Check sheet for the modelled part. Datum: model origin and axes. Units: mm. Face numbers are marked on the shaded views. A direction names the side the tool comes from. Give positions to 0.01 mm unless a question says otherwise; leave off trailing zeros. Loops run counter-clockwise (first coordinate to the right, second up) from the corner with the lowest first, then second, coordinate; pieces in that order, holes last. Notation, with made-up numbers: M 17,45 L 70,45 A16 ccw 70,71 Z; hole C 25,79.25 d1. An arc over 180 degrees is marked long. One line per question, with ' | ' between items. Start each with the question number.
from build123d import *

# Parameters (mm, degrees)
SKETCH1_W           = 30.4
SKETCH1_H           = 3.2
BOSS_EXTRUDE1_DEPTH = 17.6
SKETCH2_R           = 1.5
CUT_EXTRUDE1_DEPTH  = 16
SKETCH3_R           = 1.075
CUT_EXTRUDE2_DEPTH  = 16
SKETCH4_W           = 22.4
SKETCH4_H           = 3.2
BOSS_EXTRUDE2_DEPTH = 12.8
SKETCH5_R           = 1.075
CUT_EXTRUDE3_DEPTH  = 16
SKETCH6_W           = 14.4
SKETCH6_H           = 14.4
BOSS_EXTRUDE3_DEPTH = 3.2
SKETCH7_R           = 1.5
CUT_EXTRUDE4_DEPTH  = 59.356147919
SKETCH8_R           = 6
CUT_EXTRUDE5_DEPTH  = 3.2
FILLET5_R           = 4
FILLET6_R           = 10
FILLET7_R           = 6
FILLET8_R           = 10
FILLET9_R           = 3
FILLET10_R          = 10
FILLET12_R          = 3


# Some blends are built 0.0001 mm under size
with BuildPart() as part:
    # Sketch1 → Boss-Extrude1 (new body)
    with BuildSketch(Plane(origin=(0, 0, 0), x_dir=(1, 0, 0), z_dir=(0, 1, 0))):
        with Locations((15.2, -1.6)):
            Rectangle(SKETCH1_W, SKETCH1_H)
    extrude(amount=BOSS_EXTRUDE1_DEPTH)

    # Sketch2 → Cut-Extrude1 (cut)
    with BuildSketch(Plane.XY.offset(3.2)):
        with Locations((23.2, 6.4)):
            Circle(SKETCH2_R)
        with Locations((7.2, 6.4)):
            Circle(SKETCH2_R)
    extrude(amount=-CUT_EXTRUDE1_DEPTH, mode=Mode.SUBTRACT)

    # Sketch3 → Cut-Extrude2 (cut)
    with BuildSketch(Plane(origin=(0, 0, 0), x_dir=(-1, 0, 0), z_dir=(0, 0, -1))):
        with Locations((-27.2, 12.8)):
            Circle(SKETCH3_R)
        with Locations((-3.2, 12.8)):
            Circle(SKETCH3_R)
    extrude(amount=-CUT_EXTRUDE2_DEPTH, mode=Mode.SUBTRACT)

    # Sketch4 → Boss-Extrude2 (add)
    with BuildSketch(Plane(origin=(0, 17.6, 0), x_dir=(1, 0, 0), z_dir=(0, 1, 0))):
        with Locations((15.2, -1.6)):
            Rectangle(SKETCH4_W, SKETCH4_H)
    extrude(amount=BOSS_EXTRUDE2_DEPTH)

    # Sketch5 → Cut-Extrude3 (cut)
    with BuildSketch(Plane.XY.offset(3.2)):
        with Locations((12, 24)):
            Circle(SKETCH5_R)
    extrude(amount=-CUT_EXTRUDE3_DEPTH, mode=Mode.SUBTRACT)

    # Sketch6 → Boss-Extrude3 (add)
    with BuildSketch(Plane.XY.offset(3.2)):
        with Locations((-3.2, 34.4)):
            Rectangle(SKETCH6_W, SKETCH6_H)
        with Locations((33.6, 34.4)):
            Rectangle(SKETCH6_W, SKETCH6_H)
    extrude(amount=-BOSS_EXTRUDE3_DEPTH)

    # Sketch7 → Cut-Extrude4 (cut, through all)
    with BuildSketch(Plane.XY.offset(3.2)):
        with Locations((-6.725, 38.2)):
            Circle(SKETCH7_R)
        with Locations((37.125, 38.2)):
            Circle(SKETCH7_R)
    extrude(amount=-CUT_EXTRUDE4_DEPTH, mode=Mode.SUBTRACT)

    # Sketch8 → Cut-Extrude5 (cut)
    with BuildSketch(Plane.XY.offset(3.2)):
        with Locations((15.2, 35.549818305)):
            Circle(SKETCH8_R)
    extrude(amount=-CUT_EXTRUDE5_DEPTH, mode=Mode.SUBTRACT)

    # Fillet5
    fillet5_edges = [part.edges().sort_by_distance(p)[0] for p in [
        (0, 17.6, 1.6),
        (30.4, 17.6, 1.6),
    ]]
    fillet(fillet5_edges, radius=FILLET5_R - 0.0001)  # a hair under: the kernel refuses the full size

    # Fillet6
    # the kernel refuses this fillet: 10 mm, written as the material it adds along each edge
    with BuildSketch(Plane(origin=(26.4, 30.4, 3.2), x_dir=(0, 1, 0), z_dir=(0, 0, -1)), Plane(origin=(4, 30.4, 0), x_dir=(0, 1, 0), z_dir=(0, 0, 1))) as fillet6_piece_1:
        with BuildLine():
            CenterArc((9.821908657, -10), FILLET6_R, 90, 79.170567871)
            Line((0, -8.121141214), (-0.196438173, -8.083564039))
            ThreePointArc((-0.196438173, -8.083564039), (-0.2, -4.060570607), (-0.2, 0))
            Line((-0.2, 0), (0, 0.2))
            Line((0, 0.2), (9.821908657, 0.2))
            Line((9.821908657, 0.2), (9.821908657, 0))
        make_face()
    extrude(amount=3.2)

    # Fillet7
    fillet7_edges = [part.edges().sort_by_distance(p)[0] for p in [
        (4, 27.2, 1.6),
        (26.4, 27.2, 1.6),
    ]]
    fillet(fillet7_edges, radius=FILLET7_R)

    # Fillet8
    fillet8_edges = [part.edges().sort_by_distance(p)[0] for p in [
        (40.8, 27.2, 1.6),
        (-10.4, 27.2, 1.6),
    ]]
    fillet(fillet8_edges, radius=FILLET8_R)

    # Fillet9
    fillet9_edges = [part.edges().sort_by_distance(p)[0] for p in [
        (-10.4, 41.6, 1.6),
        (40.8, 41.6, 1.6),
    ]]
    fillet(fillet9_edges, radius=FILLET9_R)

    # Fillet10
    fillet10_edges = [part.edges().sort_by_distance(p)[0] for p in [
        (26.4, 41.6, 1.6),
        (4, 41.6, 1.6),
    ]]
    fillet(fillet10_edges, radius=FILLET10_R)

    # Fillet12
    fillet12_edges = [part.edges().sort_by_distance(p)[0] for p in [
        (4, 17.6, 1.6),
        (26.4, 17.6, 1.6),
    ]]
    fillet(fillet12_edges, radius=FILLET12_R)


solid = part.part
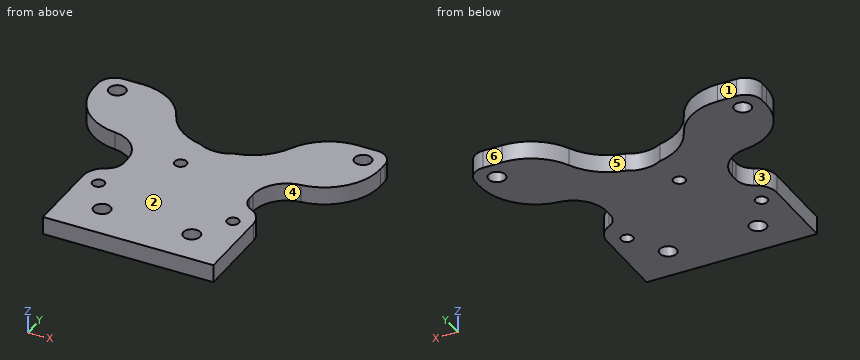
Q1. Cross-section at B-B (y = 24). Record the cut outline in (x, z) (3 decimals), and give its area (3 significant figures).
Q2. Access from +Z, -Z, +X, -X, +Y, -Y to the whole of each face (thin tool, end or side, straight path). Record for the marked faces 4, 5 and 6.
Q3. Depth check by flat-ended pin: P1, Ø1, axis at x = 10, z = 2, coming from the +Y side; P2, Ø0.6, axis at y = 20.5, z = 2.5, coming from the -X side; P3, Ø1.6, axis at y = 10, z = 1.5, coming from the -X side. Enter the tip coordinate at first touch or a pass-through.
Q4. Draft check along Y on the marked faces 1, 2 and 3. Enter one of: released by +Y, released by -Y, zero draft, split by the parting line, or undercut.
Q5. Material ranges on probe 1 along X at (y, z) = (13.5, 0.75); probe 2 along X at (y, z) = (21.5, 2.55); probe 3 along Y at (x, z) = (7, 0.4), recorded low to high. Write a range as from..to.
Q6. Cross-section at C-C (x = 23.2). Record the cut outline in (y, z).
Q7. Cross-section at A-A (y = 6.4). Record the cut outline in (x, z).
Q8. Cross-section at D-D (z = 1.45). State how many separate pieces and enclosed holes the cut face has, and give its area (3 significant figures).
Solved:
1) outline: M 3.307,0 L 10.925,0 L 10.925,3.2 L 3.307,3.2 Z; M 13.075,0 L 27.093,0 L 27.093,3.2 L 13.075,3.2 Z | area: 69.2 mm²
2) face 4: +Z, -Z, +X | face 5: +Z, -Z, +Y | face 6: +Z, -Z, +X, -X, +Y
3) P1: stops at y = 31.29 | P2: stops at x = 4 | P3: stops at x = 0
4) face 1: released by +Y | face 2: zero draft | face 3: undercut
5) probe 1: x = 0..2.38, 4.02..26.38, 28.02..30.4 | probe 2: x = 3.99..26.41 | probe 3: y = 0..4.91, 7.89..33.08
6) outline: M 0,0 L 4.9,0 L 4.9,3.2 L 0,3.2 Z; M 7.9,0 L 32.89,0 L 32.89,3.2 L 7.9,3.2 Z
7) outline: M 0,0 L 5.7,0 L 5.7,3.2 L 0,3.2 Z; M 8.7,0 L 21.7,0 L 21.7,3.2 L 8.7,3.2 Z; M 24.7,0 L 30.4,0 L 30.4,3.2 L 24.7,3.2 Z
8) separate pieces: 1 | enclosed holes: 7 | area: 1,180 mm²
